Build history of the part. All positions in model axes, mm. Face numbers are marked on the shaded views. A direction names the side the tool comes from. Round coordinates to 2 decimals unless told otherwise and drop trailing zeros. Write each loop counter-clockwise with the first axis right and the second up, starting at its lowest first coordinate (ties: lowest second). Pieces come first, ordered by that corner, then holes. Notation, with made-up numbers: (32, -38.5) -> (88, -38.5) arc R33 cw to (88, -3.5) -> close; hole circle Ø6 at (-32, 79). An arc over 180 degrees is marked (long way). Answer as CSV lines item,"result".
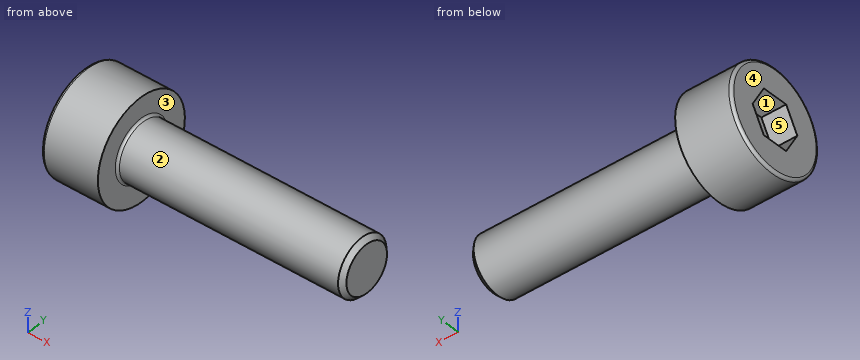
from build123d import *

# Parameters (mm, degrees)
FILLET1_R      = 0.1
FILLET2_R      = 0.12
CHAMFER1_SIZE  = 0.2
EXTRUDE1_DEPTH = 1.1


with BuildPart() as part:
    # Sketch1 → Revolve1 (revolve)
    with BuildSketch(Plane.XY, mode=Mode.PRIVATE) as revolve1_sk:
        Polygon((2.5, 1.25), (2.5, 0), (4.279914881, 0), (12.5, 0), (12.5, 1.25), align=None)
        Polygon((0, 2.25), (0, 0), (2.5, 0), (2.5, 1.25), (2.5, 2.25), align=None)
    revolve(revolve1_sk.sketch.rotate(Axis((0, 0, 0), (1, 0, 0)), 90), axis=Axis((0, 0, 0), (1, 0, 0)))

    # Fillet1
    fillet1_edges = [part.edges().sort_by_distance(p)[0] for p in [
        (2.5, 0, -1.25),
    ]]
    fillet(fillet1_edges, radius=FILLET1_R)

    # Fillet2
    fillet2_edges = [part.edges().sort_by_distance(p)[0] for p in [
        (0, 0, -2.25),
    ]]
    fillet(fillet2_edges, radius=FILLET2_R)

    # Chamfer1
    chamfer1_edges = [part.edges().sort_by_distance(p)[0] for p in [
        (12.5, 0, -1.25),
    ]]
    chamfer(chamfer1_edges, length=CHAMFER1_SIZE)

    # Sketch2 → Extrude1 (cut)
    with BuildSketch(Plane.ZY):
        Polygon((0, 1.154700538), (-1, 0.577350269), (-1, -0.577350269), (0, -1.154700538), (1, -0.577350269), (1, 0.577350269), align=None)
    extrude(amount=-EXTRUDE1_DEPTH, mode=Mode.SUBTRACT)


solid = part.part
1. Cut at A-A, the plane y = 0. Write the cut outline in (x, z), then the cut area to 3 significant figures.
Results found:
outline,"(0, -2.13) arc R0.12 ccw to (0.12, -2.25) -> (2.5, -2.25) -> (2.5, -1.35) arc R0.1 cw to (2.6, -1.25) -> (12.3, -1.25) -> (12.5, -1.05) -> (12.5, 1.05) -> (12.3, 1.25) -> (2.6, 1.25) arc R0.1 cw to (2.5, 1.35) -> (2.5, 2.25) -> (0.12, 2.25) arc R0.12 ccw to (0, 2.13) -> (0, 1) -> (1.1, 1) -> (1.1, -1) -> (0, -1) -> close"
area,"34.0 mm2"
2. Cut at B-B, the plane x = 9. Write the cut outline in (y, z), then the cut area to 3 significant figures.
Results found:
outline,"circle Ø2.5 at (0, 0)"
area,"4.91 mm2"
3. Mould opens along Y. For the marked faces 1, 2 and 3 say: +Y half, -Y half, draft (parallel to the pull), parting line (faces both ways), or undercut.
Results found:
face 1,"undercut"
face 2,"parting line"
face 3,"draft"
4. Drop a flat-ended pin along its axis: pin 1 Ø2 at (x, y) = (9.5, 1) entering from -Z. Give the stop position or say it passes through.
Results found:
pin 1,"stops at z = -1.25"
5. Probe line 1 along X through (y, z) = (-0.1, -2); line 2 along X through (y, z) = (-0.95, 0.3); line 3 along Y through (x, z) = (1, -0.15) (3 decimals). List the from-to ranges inside material, lowest first.
Results found:
line 1,"x = 0 to 2.5"
line 2,"x = 1.1 to 12.5"
line 3,"y = -2.245 to -1.068, 1.068 to 2.245"
6. Which spindle directions (+Z, -Z, +X, -X, +Y, -Y) get a long thin tool onto all of the face, cutting with end or side? Do the marked faces 4 and 5. Say none if no direction does.
Results found:
face 4,"+Z, -Z, -X, +Y, -Y"
face 5,"-X"
